The listing builds one solid part. Answer for the finished solid, in the listing's coordinates (mm). Round coordinates to 2 decimals unless told otherwise and drop trailing zeros. Loops run counter-clockwise (first coordinate to the right, second up) from the corner with the lowest first, then second, coordinate; pieces in that order, holes last. Notation, with made-up numbers: M 23.25,-33.5 L 55.25,-33.5 A36 cw 55.25,2.5 Z; hole C 79,-33.5 d3. An arc over 180 degrees is marked long. Answer as a JSON object with one key per item and string values.
```python
from build123d import *

# Parameters (mm, degrees)
SKETCH1_W           = 79.5
SKETCH1_H           = 55.45
SKETCH1_W_2         = 77
SKETCH1_H_2         = 52.15
BOSS_EXTRUDE1_DEPTH = 0.6
SKETCH2_W           = 81.1
SKETCH2_H           = 57.05
SKETCH2_W_2         = 76
SKETCH2_H_2         = 51.15
BOSS_EXTRUDE2_DEPTH = 0.6


with BuildPart() as part:
    # Sketch1 → Boss-Extrude1 (new body)
    with BuildSketch(Plane.XY):
        Rectangle(SKETCH1_W, SKETCH1_H)
        Rectangle(SKETCH1_W_2, SKETCH1_H_2, mode=Mode.SUBTRACT)
    extrude(amount=BOSS_EXTRUDE1_DEPTH)

    # Sketch2 → Boss-Extrude2 (add)
    with BuildSketch(Plane(origin=(0, 0, 0), x_dir=(-1, 0, 0), z_dir=(0, 0, -1))):
        Rectangle(SKETCH2_W, SKETCH2_H)
        Rectangle(SKETCH2_W_2, SKETCH2_H_2, mode=Mode.SUBTRACT)
    extrude(amount=BOSS_EXTRUDE2_DEPTH)


solid = part.part
```
Item 1: Flat-ended cylindrical pins translate along their axes: P1, Ø0.5, axis at y = 0, z = 0.5, coming from the -X side; P2, Ø17, axis at x = -19.5, y = 13.5, coming from the +Z side. Find the tip coordinate at first contact, or state that the pin passes through.
Values follow:
{"P1": "x = -39.75", "P2": "through"}
Item 2: The part is cut by section C-C (z = -0.4). Give the vertices of the cut face in (x, y) (3 decimals), then the cut area to 3 significant figures.
Values follow:
{"outline": "M -40.55,-28.525 L 40.55,-28.525 L 40.55,28.525 L -40.55,28.525 Z; hole M -38,-25.575 L 38,-25.575 L 38,25.575 L -38,25.575 Z", "area": "739 mm^2"}
Item 3: Straight lines are drawn through the part: line 1 (Y direction, x = 27, z = -0.3) (3 decimals); line 2 (X direction, y = -11, z = -0.35); line 3 (Y direction, x = 15, z = 0.1) (3 decimals). For each, find the intervals that lie inside material, in ascending order.
Values follow:
{"line 1": "-28.525 to -25.575, 25.575 to 28.525", "line 2": "-40.55 to -38, 38 to 40.55", "line 3": "-27.725 to -26.075, 26.075 to 27.725"}
Item 4: The part is cut by section B-B (x = -33.5). Give the vertices of the cut face in (y, z) (3 decimals), then the cut area to 3 significant figures.
Values follow:
{"outline": "M -28.525,-0.6 L -25.575,-0.6 L -25.575,0 L -26.075,0 L -26.075,0.6 L -27.725,0.6 L -27.725,0 L -28.525,0 Z; M 25.575,-0.6 L 28.525,-0.6 L 28.525,0 L 27.725,0 L 27.725,0.6 L 26.075,0.6 L 26.075,0 L 25.575,0 Z", "area": "5.52 mm^2"}
Item 5: The part is cut by section A-A (y = -12). Give the vertices of the cut face in (x, z).
Values follow:
{"outline": "M -40.55,-0.6 L -38,-0.6 L -38,0 L -38.5,0 L -38.5,0.6 L -39.75,0.6 L -39.75,0 L -40.55,0 Z; M 38,-0.6 L 40.55,-0.6 L 40.55,0 L 39.75,0 L 39.75,0.6 L 38.5,0.6 L 38.5,0 L 38,0 Z"}
